```python
from build123d import *

# Parameters (mm, degrees)
BOSS_EXTRUDE1_DEPTH = 1.5875
SKETCH2_R           = 4.7625
SKETCH2_R_2         = 6.35
CUT_EXTRUDE1_DEPTH  = 206.048954313
FILLET1_R           = 12.7


with BuildPart() as part:
    # Sketch1 → Boss-Extrude1 (new body)
    with BuildSketch(Plane.XY):
        with BuildLine():
            Line((-55.575312576, -162.067948142), (-47.839788583, -163.268748691))
            Line((-47.839788583, -163.268748691), (-47.839788583, -44.216449654))
            Line((-47.839788583, -44.216449654), (-124.039788583, -44.216449654))
            Line((-124.039788583, -44.216449654), (-118.722269766, -94.836839988))
            add(Edge.make_bspline(
                [(-55.575312576, -162.067948142), (-55.59376342, -162.065079619), (-55.650171893, -162.056309885), (-55.85836741, -162.023649386), (-56.351423804, -161.94437151), (-57.298183962, -161.782953677), (-59.601702252, -161.351219818), (-62.636225688, -160.651117849), (-66.258238647, -159.610029405), (-69.466373553, -158.528422888), (-72.693657497, -157.269325681), (-75.860283712, -155.860035916), (-78.959504505, -154.303585309), (-81.9847211, -152.603319472), (-84.929496882, -150.762889625), (-87.787571241, -148.786244312), (-90.552872427, -146.677620258), (-93.219530166, -144.441532812), (-95.781887647, -142.082765831), (-98.23451307, -139.606361101), (-100.572210643, -137.017607297), (-102.790031074, -134.322028508), (-104.883281533, -131.525372358), (-106.847535073, -128.633597727), (-108.67863952, -125.652862104), (-110.372725796, -122.589508584), (-111.926215689, -119.450052525), (-113.33582904, -116.24116789), (-114.598590351, -112.969673286), (-115.711834779, -109.642517734), (-116.673213527, -106.266766169), (-117.480698597, -102.849584725), (-118.13258691, -99.398225801), (-118.490033874, -96.886133888), (-118.655606827, -95.451511305), (-118.689766491, -95.14113961), (-118.706492882, -94.98591445), (-118.715898664, -94.897412794), (-118.721125626, -94.847717815), (-118.722269766, -94.836839988)],
                knots=[0, 0, 0, 0, 0.000570634, 0.001744558, 0.006440232, 0.015831442, 0.031091736, 0.078042667, 0.110904268, 0.146108785, 0.181308268, 0.216502219, 0.251690199, 0.286871835, 0.322046819, 0.357214911, 0.392375937, 0.427529794, 0.462676442, 0.497815906, 0.532948271, 0.568073682, 0.603192339, 0.638304491, 0.673410436, 0.708510515, 0.743605108, 0.77869463, 0.813779526, 0.84886027, 0.88393736, 0.919011312, 0.954082662, 0.989151956, 0.994996677, 0.997334555, 0.998503491, 0.999672426, 1, 1, 1, 1], degree=3))
        make_face()
    extrude(amount=BOSS_EXTRUDE1_DEPTH)

    # Sketch2 → Cut-Extrude1 (cut, through all)
    with BuildSketch(Plane(origin=(0, 0, 0), x_dir=(-1, 0, 0), z_dir=(0, 0, -1))):
        with Locations((64.349788583, -118.511449654)):
            Circle(SKETCH2_R)
        with Locations((85.939788583, -118.511449654)):
            Circle(SKETCH2_R)
        with Locations((73.239788583, -93.111449654)):
            Circle(SKETCH2_R_2)
        with Locations((98.639788583, -93.111449654)):
            Circle(SKETCH2_R_2)
        with Locations((98.639788583, -64.536449654)):
            Circle(SKETCH2_R_2)
        with Locations((73.239788583, -64.536449654)):
            Circle(SKETCH2_R_2)
    extrude(amount=-CUT_EXTRUDE1_DEPTH, mode=Mode.SUBTRACT)

    # Fillet1
    fillet1_edges = [part.edges().sort_by_distance(p)[0] for p in [
        (-47.839788583, -44.216449654, 0.79375),
        (-47.839788583, -163.268748691, 0.79375),
    ]]
    fillet(fillet1_edges, radius=FILLET1_R)


solid = part.part
```
Model file for the job. Use its own axes, mm. Round coordinates to 2 decimals unless told otherwise and drop trailing zeros. Write each loop counter-clockwise with the first axis right and the second up, starting at its lowest first coordinate (ties: lowest second). Pieces come first, ordered by that corner, then holes. Notation, with made-up numbers: M 57,68 L 106,68 A7 cw 106,73 Z; hole C -21.5,3 d3. An arc over 180 degrees is marked long. Put each result on its own line as item: value.
Item 1: Cut at A-A (y = -89). List the corners of the cut face in (x, z), and give its area (3 significant figures).
Responses:
outline: M -119.34,0 L -103.48,0 L -103.48,1.59 L -119.34,1.59 Z; M -93.8,0 L -78.08,0 L -78.08,1.59 L -93.8,1.59 Z; M -68.4,0 L -47.84,0 L -47.84,1.59 L -68.4,1.59 Z
area: 82.8 mm²
Item 2: Mould opens along X. For faces 1 (the cylindrical face through (-85.32, -113.79, 0.78)), 2 (the cylindrical face through (-51.461, -48.035, 0.805)), 3 (the flat face through (-78, -102, 1.588)) say: +X half, -X half, draft (parallel to the pull), parting line (faces both ways), or undercut.
Responses:
face 1: undercut
face 2: +X half
face 3: draft
Item 3: Flat gauge pin, fed straight in: P1, Ø8, axis at x = -64, y = -62, coming from the -Z side. Where does the tip first touch, or does it go through?
Responses:
P1: z = 0
Item 4: Cut at B-B (x = -73). State how many separate pieces and enclosed holes the cut face has, and give its area (3 significant figures).
Responses:
separate pieces: 3
enclosed holes: 0
area: 139 mm²
Item 5: Probe L1, parallel to Y at x = -96, z = 0.65; L2, parallel to Y at x = -73, z = 0.7; L3, parallel to X at y = -116.5, z = 0.55. List the from-to ranges inside material, lowest first. Write a range as from..to.
Responses:
L1: -141.83..-98.89, -87.34..-70.31, -58.76..-44.22
L2: -157.11..-99.46, -86.77..-70.88, -58.19..-44.22
L3: -113.2..-90.26, -81.62..-68.67, -60.03..-47.84
